Design review of the part built by this model. Coordinates are the model's own, in mm. Coordinates: 2 decimals unless noted, no trailing zeros. Loops run counter-clockwise (first coordinate to the right, second up) from the corner with the lowest first, then second, coordinate; pieces in that order, holes last. Notation, with made-up numbers: (-9, 64) -> (46, 64) arc R18 ccw to (46, 82) -> close; hole circle Ø1 at (52, -8). An arc over 180 degrees is marked (long way). Use a Markdown table: item, result. Add a question column.
Q1. For probe 1 along Y at (x, z) = (0, 0.3); probe 2 along Z at (x, y) = (1.75, -0.75); probe 3 along Y at (x, z) = (0, 0.8), list the stretches that pass through material, from the lowest coordinate up.
Q2. Clearance check with flat-ended pins moving along their axes: pin 1 Ø1.8 at (x, y) = (0, 0) entering from +Z; pin 2 Ø1 at (y, z) = (1.5, 1.5) entering from -X. State where each tip first meets the part, or that it passes through.
Q3. Take a section at C-C on z = 0.55. Write out the cut boundary in (x, y).
Q4. Draft analysis for pull direction Y (two halves, no side actions). For faces 1 (the face through (-3, 0.1, 0.2)), 2 (the face through (1.3, 0, 0)), 3 (the face through (1.05, 0.33, 0.49)), state which applies: pulls with the +Y half, pulls with the -Y half, needs draft (parallel to the pull), parting line crosses it, or undercut.
Q5. Take a section at A-A on x = 0. Write out the cut boundary in (y, z).
Q6. Take a section at B-B on z = 0.2. Write out the cut boundary in (x, y), plus the area to 3 significant figures.
from build123d import *

# Parameters (mm, degrees)
F7_R  = 3
F8_R  = 3
F10_R = 2.2
F9_R  = 1.95
F11_R = 1.95
F13_R = 1.1
F12_R = 1.1


with BuildPart() as f14:
    # F7 (on Top) → F14 section 0
    with BuildSketch(Plane.XY):
        Circle(F7_R)
    # F8 (on offset) → F14 section 1
    with BuildSketch(Plane.XY.offset(0.35)):
        Circle(F8_R)
    loft()

    # F10 (on offset) → F15 section 0
    with BuildSketch(Plane.XY.offset(2)):
        Circle(F10_R)
    # F8 (on offset) → F15 section 1
    with BuildSketch(Plane.XY.offset(0.35)):
        Circle(F8_R)
    loft()

    # F9 (on offset) → F16 section 0
    with BuildSketch(Plane.XY.offset(2)):
        Circle(F9_R)
    # F11 (on offset) → F16 section 1
    with BuildSketch(Plane.XY.offset(1)):
        Circle(F11_R)
    loft(mode=Mode.SUBTRACT)

    # F13 (on offset) → F17 section 0
    with BuildSketch(Plane.XY.offset(1)):
        Circle(F13_R)
    # F12 (on Top) → F17 section 1
    with BuildSketch(Plane.XY):
        Circle(F12_R)
    loft(mode=Mode.SUBTRACT)


solid = f14.part
Answer list:
| question | item | result |
|---|---|---|
| 1 | probe 1 | -3 to -1.1, 1.1 to 3 |
| 1 | probe 2 | 0 to 1 |
| 1 | probe 3 | -2.78 to -1.1, 1.1 to 2.78 |
| 2 | pin 1 | through |
| 2 | pin 2 | x = -2.35 |
| 3 | outline | circle Ø5.81 at (0, 0); hole circle Ø2.2 at (0, 0) |
| 4 | face 1 | parting line crosses it |
| 4 | face 2 | needs draft |
| 4 | face 3 | undercut |
| 5 | outline | (-3, 0) -> (-1.1, 0) -> (-1.1, 1) -> (-1.95, 1) -> (-1.95, 2) -> (-2.2, 2) -> (-3, 0.35) -> close; (1.1, 0) -> (3, 0) -> (3, 0.35) -> (2.2, 2) -> (1.95, 2) -> (1.95, 1) -> (1.1, 1) -> close |
| 6 | outline | circle Ø6 at (0, 0); hole circle Ø2.2 at (0, 0) |
| 6 | area | 24.5 mm² |
